Answer from the drawing. Dimensions are ordinates in mm from the lowest x, y and z of the part. Round coordinates to 2 decimals unless told otherwise and drop trailing zeros. Loops run counter-clockwise (first coordinate to the right, second up) from the corner with the lowest first, then second, coordinate; pieces in that order, holes last. Notation, with made-up numbers: (51, 81) - (77, 81) arc R18 cw to (77, 86) - close; hole circle Ø10 at (80, 45). An arc over 180 degrees is marked (long way). Return JSON: item names as keys, results as strings.
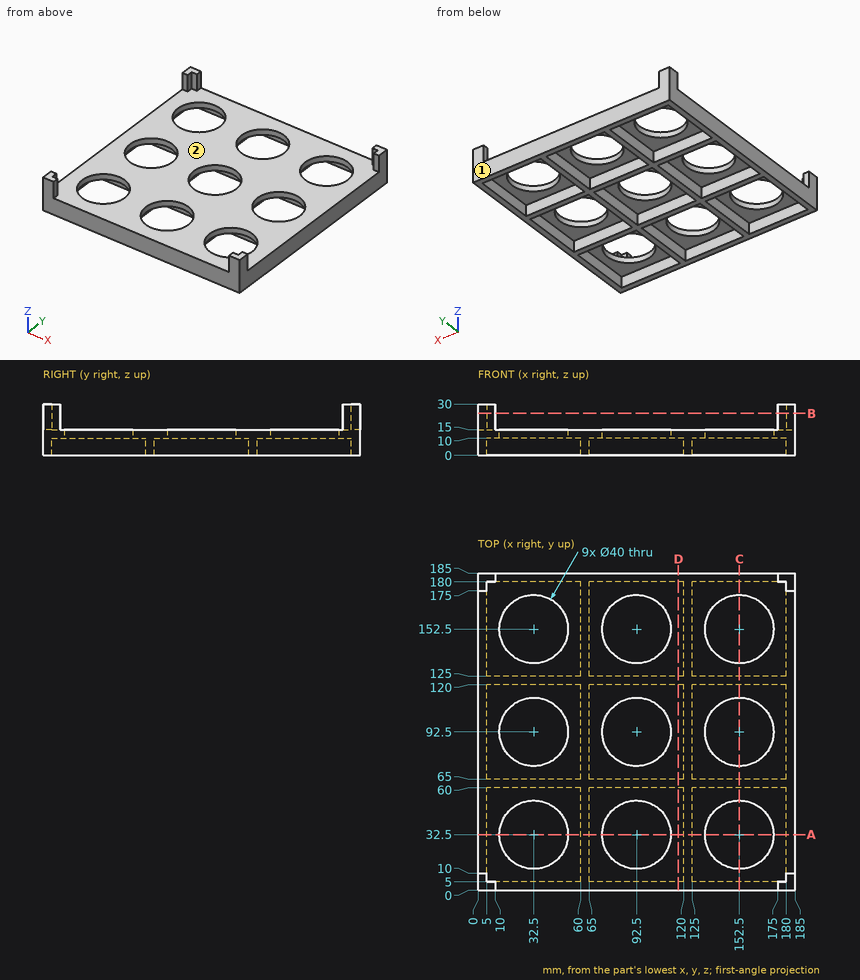
1) Section A-A (y = 32.5) is taken. Give the vertices of the cut face in (x, z), and give its area (3 significant figures).
Verdict:
{"outline": "(0, 0) - (5, 0) - (5, 10) - (12.5, 10) - (12.5, 15) - (0, 15) - close; (52.5, 10) - (60, 10) - (60, 0) - (65, 0) - (65, 10) - (72.5, 10) - (72.5, 15) - (52.5, 15) - close; (112.5, 10) - (120, 10) - (120, 0) - (125, 0) - (125, 10) - (132.5, 10) - (132.5, 15) - (112.5, 15) - close; (172.5, 10) - (180, 10) - (180, 0) - (185, 0) - (185, 15) - (172.5, 15) - close", "area": "525 mm2"}
2) Find the intervals of material crossed by L1, parallel to Y at x = 152.5, z = 13.8; L2, parallel to X at y = 41.5, z = 4.5, in increasing order.
Verdict:
{"L1": "y = 0 to 12.5, 52.5 to 72.5, 112.5 to 132.5, 172.5 to 185", "L2": "x = 0 to 5, 60 to 65, 120 to 125, 180 to 185"}
3) Flat-ended cylindrical pins translate along their axes: pin 1 (8 mm diameter, centred on y = 73.5, z = 19.5, fed in from -X); pin 2 (3 mm diameter, centred on x = 32.5, y = 69, fed in from +Z). Find the tip coordinate at first contact, or state that the pin passes through.
Verdict:
{"pin 1": "passes through", "pin 2": "stops at z = 15"}
4) Section D-D (x = 117) is taken. Give the vertices of the cut face in (y, z).
Verdict:
{"outline": "(0, 0) - (5, 0) - (5, 10) - (60, 10) - (60, 0) - (65, 0) - (65, 10) - (120, 10) - (120, 0) - (125, 0) - (125, 10) - (180, 10) - (180, 0) - (185, 0) - (185, 15) - (0, 15) - close"}
5) Determine the mould class of the marked faces 1 and 2 for opening direction X: pulls with the +X half, pulls with the -X half, needs draft (parallel to the pull), parting line crosses it, or undercut.
Verdict:
{"face 1": "needs draft", "face 2": "undercut"}
6) Section B-B (z = 24.5) is taken. Give the vertices of the cut face in (x, y), and give its area (3 significant figures).
Verdict:
{"outline": "(0, 0) - (10, 0) - (10, 5) - (5, 5) - (5, 10) - (0, 10) - close; (0, 175) - (5, 175) - (5, 180) - (10, 180) - (10, 185) - (0, 185) - close; (175, 0) - (185, 0) - (185, 10) - (180, 10) - (180, 5) - (175, 5) - close; (175, 180) - (180, 180) - (180, 175) - (185, 175) - (185, 185) - (175, 185) - close", "area": "300 mm2"}
